Design review of the part built by this model. Coordinates are the model's own, in mm. Face numbers are marked on the shaded views. A direction names the side the tool comes from. Give positions to 0.01 mm unless a question says otherwise; leave off trailing zeros. Write each loop counter-clockwise with the first axis right and the second up, starting at its lowest first coordinate (ties: lowest second). Pieces come first, ordered by that corner, then holes.
```python
from build123d import *

# Parameters (mm, degrees)
BOSS_EXTRUDE1_DEPTH = 12
SKETCH3_R           = 2
BOSS_EXTRUDE2_DEPTH = 1
FILLET3_R           = 1
BOSS_EXTRUDE3_START = 0.5
SKETCH4_R           = 2
BOSS_EXTRUDE3_DEPTH = 0.5
SKETCH5_R           = 0.25
CUT_EXTRUDE1_DEPTH  = 0.25
SKETCH6_R           = 0.25
BOSS_EXTRUDE4_DEPTH = 2.5
SKETCH7_R           = 1.5
BOSS_EXTRUDE5_DEPTH = 2
CUT_EXTRUDE11_DEPTH = 2
CIRPATTERN2_COUNT   = 12


with BuildPart() as part:
    # Sketch2 → Boss-Extrude1 (new body)
    with BuildSketch(Plane(origin=(0, 0, 0), x_dir=(1, 0, 0), z_dir=(0, 1, 0))):
        with BuildLine():
            Line((-3, 4), (3, 4))
            ThreePointArc((3, 4), (5, 0), (3, -4))
            Line((3, -4), (-3, -4))
            ThreePointArc((-3, -4), (-5, 0), (-3, 4))
        make_face()
    extrude(amount=BOSS_EXTRUDE1_DEPTH)

    # Sketch3 → Boss-Extrude2 (add)
    with BuildSketch(Plane(origin=(0, 0, 0), x_dir=(-1, 0, 0), z_dir=(0, -1, 0))):
        with Locations(Location((0, 0, 0), (0, 0, 90))):
            Circle(SKETCH3_R)
    extrude(amount=BOSS_EXTRUDE2_DEPTH)

    # Fillet3
    fillet3_edges = [part.edges().sort_by_distance(p)[0] for p in [
        (-3, 6, -4),
        (3, 6, -4),
        (3, 6, 4),
        (-3, 6, 4),
    ]]
    fillet(fillet3_edges, radius=FILLET3_R)

    # Sketch4 → Boss-Extrude3 (add)
    with BuildSketch(Plane(origin=(0, 12, 0), x_dir=(1, 0, 0), z_dir=(0, 1, 0)).offset(BOSS_EXTRUDE3_START)):
        with Locations(Location((0, 0, 0), (0, 0, 90))):
            Circle(SKETCH4_R)
    extrude(amount=-BOSS_EXTRUDE3_DEPTH)

    # Sketch5 → Cut-Extrude1 (cut)
    with BuildSketch(Plane(origin=(0, 12, 0), x_dir=(1, 0, 0), z_dir=(0, 1, 0))):
        with Locations(Location((3.5, 0, 0), (0, 0, 270))):
            Circle(SKETCH5_R)
    cut_extrude1 = extrude(amount=-CUT_EXTRUDE1_DEPTH, mode=Mode.SUBTRACT)

    # Mirror1: Cut-Extrude1 across plane
    add(cut_extrude1.mirror(Plane(origin=(0, 0, 0), x_dir=(0, 0, 1), z_dir=(1, 0, 0))), mode=Mode.SUBTRACT)

    # Sketch6 → Boss-Extrude4 (add)
    with BuildSketch(Plane(origin=(0, 12.5, 0), x_dir=(1, 0, 0), z_dir=(0, 1, 0))):
        with Locations(Location((0, 0, 0), (0, 0, 270))):
            Circle(SKETCH6_R)
    extrude(amount=BOSS_EXTRUDE4_DEPTH)

    # Sketch7 → Boss-Extrude5 (add)
    with BuildSketch(Plane(origin=(0, 15, 0), x_dir=(1, 0, 0), z_dir=(0, 1, 0))):
        with Locations(Location((0, 0, 0), (0, 0, 270))):
            Circle(SKETCH7_R)
    extrude(amount=-BOSS_EXTRUDE5_DEPTH)

    # Sketch9 → Cut-Extrude11 (cut)
    with BuildSketch(Plane(origin=(0, 15, 0), x_dir=(1, 0, 0), z_dir=(0, 1, 0))):
        Polygon((-0.342020143, -0.939692621), (-0.173648178, -0.984807753), (0, -1.556082509), (-0.781544676, -1.353675088), align=None)
    cut_extrude11 = extrude(amount=-CUT_EXTRUDE11_DEPTH, mode=Mode.SUBTRACT)

    # CirPattern2: Cut-Extrude11 ×12 about axis
    cirpattern2_axis = Axis((0, 0, 0), (0, 1, 0))
    for i in range(1, CIRPATTERN2_COUNT):
        add(cut_extrude11.rotate(cirpattern2_axis, i * 360 / CIRPATTERN2_COUNT), mode=Mode.SUBTRACT)


solid = part.part
```
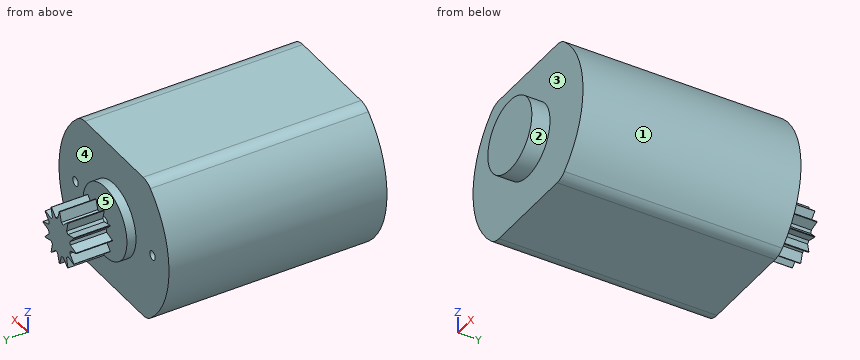
(1) Mouldability with a two-part tool opening along Y and no side actions: class the marked faces 3, 4 and 5 as pulls with the +Y half, pulls with the -Y half, needs draft (parallel to the pull), parting line crosses it, or undercut.
Resolved:
face 3: pulls with the -Y half
face 4: pulls with the +Y half
face 5: undercut
(2) To check wall thickness, follow L1, parallel to X at y = 11.9, z = 0; L2, parallel to Y at x = 2.75, z = 2; L3, parallel to X at y = 10.25, z = -3. State the ranges of each line that lie inside material, in increasing order.
Resolved:
L1: x = -5 to -3.75, -3.25 to 3.25, 3.75 to 5
L2: y = 0 to 12
L3: x = -4 to 4
(3) Tool access review of the marked faces 1 and 2: name each direction out of +Z, -Z, +X, -X, +Y, -Y from which nothing blocks a thin tool from reaching the whole face with its end or side.
Resolved:
face 1: +X, +Y, -Y
face 2: -Y
(4) Clearance check with a flat-ended pin moving along its axis: P1, Ø0.6, axis at x = 3.5, z = 0, coming from the +Y side. State where the tip first meets the part, or that it passes through.
Resolved:
P1: stops at y = 12
(5) Consider section A-A, the plane y = 10.25. Give the boundary of the cut face in (x, z), then the cut area to 3 significant figures.
Resolved:
outline: (-3.31, -3.75) arc R1 ccw to (-2.65, -4) - (2.65, -4) arc R1 ccw to (3.31, -3.75) arc R5 ccw to (3.31, 3.75) arc R1 ccw to (2.65, 4) - (-2.65, 4) arc R1 ccw to (-3.31, 3.75) arc R5 ccw to start
area: 70.3 mm2
(6) Consider section C-C, the plane x = 2.25. Give the boundary of the cut face in (y, z), then the cut area to 3 significant figures.
Resolved:
outline: (0, -4) - (12, -4) - (12, 4) - (0, 4) - close
area: 96.0 mm2
(7) Consider section D-D, the plane z = 3. Give the boundary of the cut face in (x, y).
Resolved:
outline: (-4, 0) - (4, 0) - (4, 12) - (-4, 12) - close
(8) Consider section B-B, the plane z = 1.75. Give the boundary of the cut face in (x, y).
Resolved:
outline: (-4.68, 0) - (-0.97, 0) - (-0.97, -1) - (0.97, -1) - (0.97, 0) - (4.68, 0) - (4.68, 12) - (0.97, 12) - (0.97, 12.5) - (-0.97, 12.5) - (-0.97, 12) - (-4.68, 12) - close
